Here's how the part is built. I have some questions about the finished solid (model axes, mm). Face numbers are marked on the shaded views. A direction names the side the tool comes from. Coordinates: 2 decimals unless noted, no trailing zeros. Write each loop counter-clockwise with the first axis right and the second up, starting at its lowest first coordinate (ties: lowest second). Pieces come first, ordered by that corner, then holes.
Item 1: If we section it at D-D (z = 5): Please give me the cut outline in (x, y).
Item 2: I'm going to push flat-ended pins straight in: pin 1 Ø8 at (x, y) = (6, -4) entering from +Z; pin 2 Ø2 at (y, z) = (1, 4.5) entering from -X. Where does each tip first touch, or does it pass through?
Item 3: For the marked faces 1 and 2, which set-ups out of +Z, -Z, +X, -X, +Y, -Y let a thin tool reach every point of the face, with its end or its side?
Item 4: If we section it at C-C (z = 6.5): Please give me the cut outline in (x, y), then the cut area to 3 significant figures.
Item 5: If I drill on line 1 (Z direction, x = 4, y = 8); line 2 (Z direction, x = 0.75, y = 4.25); line 3 (X direction, y = -2.25, z = 2.75), over which ranges is the centre line in solid material (lowest first)?
from build123d import *

# Parameters (mm, degrees)
F0_R     = 10
F1_DEPTH = 2
F2_R     = 5
F3_DEPTH = 4
F4_SIZE  = 0.5
F5_R     = 0.99999
F6_R     = 2.5
F7_DEPTH = 3


# Not quite as in the source:
# - a fillet or chamfer is up to 0.001 mm smaller than in the source, because OpenCascade refuses the exact size


with BuildPart() as f1:
    # F0 (on Top) → F1 (new body)
    with BuildSketch(Plane.XY):
        Circle(F0_R)
    extrude(amount=F1_DEPTH)

    # F2 (on face) → F3 (join)
    with BuildSketch(Plane.XY.offset(2)):
        Circle(F2_R)
    extrude(amount=F3_DEPTH)

    # F4
    f4_edges = [f1.edges().sort_by_distance(p)[0] for p in [
        (-5, 0, 6),
    ]]
    chamfer(f4_edges, length=F4_SIZE)

    # F5 (radius 1 in the source; OpenCascade refuses exactly that, so slightly less here)
    f5_edges = [f1.edges().sort_by_distance(p)[0] for p in [
        (-10, 0, 0),
        (-10, 0, 2),
    ]]
    fillet(f5_edges, radius=F5_R)

    # F6 (on face) → F7 (join)
    with BuildSketch(Plane.XY.offset(6)):
        Circle(F6_R)
    extrude(amount=F7_DEPTH)


solid = f1.part
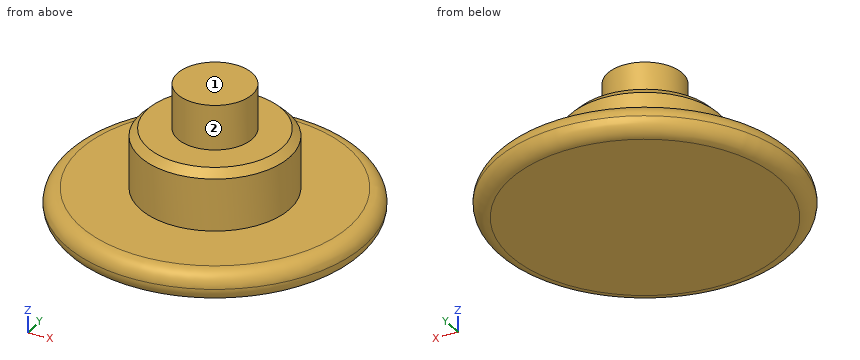
Answer list:
1. outline: circle Ø10 at (0, 0)
2. pin 1: stops at z = 6
2. pin 2: stops at x = -5
3. face 1: +Z, +X, -X, +Y, -Y
3. face 2: +Z
4. outline: circle Ø5 at (0, 0)
4. area: 19.6 mm2
5. line 1: z = 0 to 2
5. line 2: z = 0 to 6
5. line 3: x = -4.47 to 4.47
